from build123d import *

# Parameters (mm, degrees)
SKETCH_W          = 62
SKETCH_H          = 28
PAD_DEPTH         = 2
SKETCH001_W       = 57.8
SKETCH001_H       = 23.8
SKETCH001_W_2     = 53.8
SKETCH001_H_2     = 19.8
PAD001_DEPTH      = 4
SKETCH002_W       = 2
SKETCH002_H       = 23.8
PAD002_DEPTH      = 10
SKETCH003_R       = 1
POCKET_DEPTH      = 31.001
POCKET_DEPTH_BACK = -31.001
FILLET_R          = 2


with BuildPart() as part:
    # Sketch → Pad (new body)
    with BuildSketch(Plane.XY):
        Rectangle(SKETCH_W, SKETCH_H)
    extrude(amount=PAD_DEPTH)

    # Sketch001 → Pad001 (join)
    with BuildSketch(Plane.XY):
        Rectangle(SKETCH001_W, SKETCH001_H)
        Rectangle(SKETCH001_W_2, SKETCH001_H_2, mode=Mode.SUBTRACT)
    extrude(amount=PAD001_DEPTH)

    # Sketch002 → Pad002 (join)
    with BuildSketch(Plane.XY):
        with Locations((-27.9, 0)):
            Rectangle(SKETCH002_W, SKETCH002_H)
        with Locations((27.9, 0)):
            Rectangle(SKETCH002_W, SKETCH002_H)
    extrude(amount=PAD002_DEPTH)

    # Sketch003 → Pocket (cut, two sides)
    with BuildSketch(Plane.YZ) as pocket_sk:
        with Locations((0, 6)):
            Circle(SKETCH003_R)
    extrude(amount=-POCKET_DEPTH, mode=Mode.SUBTRACT)
    extrude(pocket_sk.sketch, amount=-POCKET_DEPTH_BACK, mode=Mode.SUBTRACT)

    # Fillet
    fillet_edges = [part.edges().sort_by_distance(p)[0] for p in [
        (31, 14, 1),
        (31, -14, 1),
        (-31, 14, 1),
        (-31, -14, 1),
    ]]
    fillet(fillet_edges, radius=FILLET_R)


solid = part.part
Check sheet for the modelled part. Datum: model origin and axes. Units: mm. A direction names the side the tool comes from. Round coordinates to 2 decimals unless told otherwise and drop trailing zeros. Write each loop counter-clockwise with the first axis right and the second up, starting at its lowest first coordinate (ties: lowest second). Pieces come first, ordered by that corner, then holes. Notation, with made-up numbers: (40, 52.5) - (51, 52.5) arc R34 ccw to (51, 87.5) - close; hole circle Ø11 at (-30.75, -17.5). An arc over 180 degrees is marked (long way). Return JSON: item names as keys, results as strings.
Q1. Cross-section at C-C (z = 8.75). Record the boundary of the cut face in (x, y), then the cut area to 3 significant figures.
Returned:
{"outline": "(-28.9, -11.9) - (-26.9, -11.9) - (-26.9, 11.9) - (-28.9, 11.9) - close; (26.9, -11.9) - (28.9, -11.9) - (28.9, 11.9) - (26.9, 11.9) - close", "area": "95.2 mm²"}
Q2. Cross-section at A-A (y = 0). Record the boundary of the cut face in (x, z), then the cut area to 3 significant figures.
Returned:
{"outline": "(-31, 0) - (31, 0) - (31, 2) - (28.9, 2) - (28.9, 5) - (26.9, 5) - (26.9, 2) - (-26.9, 2) - (-26.9, 5) - (-28.9, 5) - (-28.9, 2) - (-31, 2) - close; (-28.9, 7) - (-26.9, 7) - (-26.9, 10) - (-28.9, 10) - close; (26.9, 7) - (28.9, 7) - (28.9, 10) - (26.9, 10) - close", "area": "148 mm²"}
Q3. Cross-section at D-D (x = -18). Record the boundary of the cut face in (y, z), then the cut area to 3 significant figures.
Returned:
{"outline": "(-14, 0) - (14, 0) - (14, 2) - (11.9, 2) - (11.9, 4) - (9.9, 4) - (9.9, 2) - (-9.9, 2) - (-9.9, 4) - (-11.9, 4) - (-11.9, 2) - (-14, 2) - close", "area": "64.0 mm²"}
Q4. Depth check by flat-ended pin: P1, Ø2.5, axis at y = -4, z = 7, coming from the -X side; P2, Ø2.5, axis at x = 0, z = 6, coming from the -Y side; P3, Ø1, axis at x = 4, y = -7, coming from the +Z side; P4, Ø0.6, axis at x = -2, z = 3.5, coming from the -Y side. Enter the tip coordinate at first touch or a pass-through.
Returned:
{"P1": "stops at x = -28.9", "P2": "passes through", "P3": "stops at z = 2", "P4": "stops at y = -11.9"}
Q5. Scan lines: L1, parallel to X at y = -6.25, z = 2.75; L2, parallel to Z at x = -28.05, y = 0; L3, parallel to Y at x = 27.7, z = 6. Record each from-to range of solid material in increasing order. Write a range as from..to.
Returned:
{"L1": "x = -28.9..-26.9, 26.9..28.9", "L2": "z = 0..5, 7..10", "L3": "y = -11.9..-1, 1..11.9"}
Q6. Cross-section at B-B (z = 2.75). Record the boundary of the cut face in (x, y), then the cut area to 3 significant figures.
Returned:
{"outline": "(-28.9, -11.9) - (28.9, -11.9) - (28.9, 11.9) - (-28.9, 11.9) - close; hole (-26.9, -9.9) - (26.9, -9.9) - (26.9, 9.9) - (-26.9, 9.9) - close", "area": "310 mm²"}
Q7. Access from +Z, -Z, +X, -X, +Y, -Y to the whole of each face (thin tool, end or side, straight path). Record for faces 5 (the flat face through (-0.1, 11.9, 3.6)), 6 (the flat face through (28.9, 0, 4)), 7 (the flat face through (0, 11, 4)).
Returned:
{"face 5": "+Z, +X, -X, +Y", "face 6": "+Z, +X, +Y, -Y", "face 7": "+Z, +Y, -Y"}
Q8. Draft check along X on faces 1 (the cylindrical face through (30.43, 13.4, 1.01)), 2 (the flat face through (-0.1, -11.9, 3.6)), 3 (the cylindrical face through (-30.43, -13.4, 1.01)), 4 (the flat face through (0, -9.9, 3)). Enter one of: released by +X, released by -X, zero draft, split by the parting line, or undercut.
Returned:
{"face 1": "released by +X", "face 2": "zero draft", "face 3": "released by -X", "face 4": "undercut"}
